The model under review builds one solid part; all positions refer to its coordinate system, in mm. A direction names the side the tool comes from. Round coordinates to 2 decimals unless told otherwise and drop trailing zeros. Write each loop counter-clockwise with the first axis right and the second up, starting at its lowest first coordinate (ties: lowest second). Pieces come first, ordered by that corner, then holes.
Item 1: Add section B-B (y = -18). State how many separate pieces and enclosed holes the cut face has, plus the area to 3 significant figures.
Item 2: Draft analysis for pull direction Z (two halves, no side actions). For faces 4 (the face through (129, 0, -48)), 5 (the face through (124.472, -12.522, -24.842)), 6 (the face through (129, -13, 0)), state which applies: +Z half, -Z half, draft (parallel to the pull), parting line (faces both ways), or undercut.
Item 3: To check wall thickness, follow L1, parallel to Z at x = 81.28, y = -17.5; L2, parallel to X at y = -2, z = -75.5; L3, parallel to X at y = -10.25, z = -74. State the ranges of each line that lie inside material, in increasing order.
Item 4: Clearance check with flat-ended pins moving along their axes: pin 1 Ø11 at (y, z) = (-16, -8) entering from +X; pin 2 Ø10 at (y, z) = (-3.5, -28.5) entering from -X; pin 3 Ø2 at (y, z) = (-18.5, -60.5) entering from +X. State where each tip first meets the part, or that it passes through.
Item 5: Machinability: for faces 1 (the face through (254, -13, -48)), 2 (the face through (254, -13, -7)), 3 (the face through (124.472, -12.522, -69.292)), which of the approach directions +Z, -Z, +X, -X, +Y, -Y give a long, thin tool a straight path to every point of the face, cutting with its end or side? Answer none if there is none.
Item 6: Add section A-A (x = 25.4). Give the boundary of the cut face in (y, z).
Item 7: Add section C-C (z = -31.5). Give the boundary of the cut face in (x, y).
Item 8: Add section D-D (z = -97). Give the boundary of the cut face in (x, y), plus the area to 3 significant figures.
```python
from build123d import *

# Parameters (mm, degrees)
F0_R     = 12.7
F1_DEPTH = 25.4


with BuildPart() as f1:
    # F0 (on Front) → F1 (new body)
    with BuildSketch(Plane.XZ):
        with BuildLine():
            Line((254, 0), (0, 0))
            Line((0, 0), (0, -127))
            Line((0, -127), (25.4, -127))
            Line((25.4, -127), (81.28, -127))
            Line((81.28, -127), (137.16, -127))
            Line((137.16, -127), (193.04, -127))
            Line((193.04, -127), (248.92, -127))
            ThreePointArc((248.92, -127), (236.4878898258, -111.7052675251), (254, -102.6602577348))
            Line((254, -102.6602577348), (254, -81.4897422652))
            ThreePointArc((254, -81.4897422652), (236.22, -69.85), (254, -58.2102577348))
            Line((254, -58.2102577348), (254, -37.0397422652))
            ThreePointArc((254, -37.0397422652), (236.22, -25.4), (254, -13.7602577348))
            Line((254, -13.7602577348), (254, 0))
        make_face()
        with BuildLine():
            ThreePointArc((38.1, -114.3), (34.3802561211, -123.2802561211), (25.4, -127))
            ThreePointArc((25.4, -127), (16.4197438789, -105.3197438789), (38.1, -114.3))
        make_face(mode=Mode.SUBTRACT)
        with BuildLine():
            ThreePointArc((93.98, -114.3), (90.2602561211, -123.2802561211), (81.28, -127))
            ThreePointArc((81.28, -127), (72.2997438789, -105.3197438789), (93.98, -114.3))
        make_face(mode=Mode.SUBTRACT)
        with Locations((25.4, -69.85)):
            Circle(F0_R, mode=Mode.SUBTRACT)
        with Locations((81.28, -69.85)):
            Circle(F0_R, mode=Mode.SUBTRACT)
        with BuildLine():
            ThreePointArc((149.86, -114.3), (146.1402561211, -123.2802561211), (137.16, -127))
            ThreePointArc((137.16, -127), (128.1797438789, -105.3197438789), (149.86, -114.3))
        make_face(mode=Mode.SUBTRACT)
        with BuildLine():
            ThreePointArc((205.74, -114.3), (202.0202561211, -123.2802561211), (193.04, -127))
            ThreePointArc((193.04, -127), (184.0597438789, -105.3197438789), (205.74, -114.3))
        make_face(mode=Mode.SUBTRACT)
        with Locations((137.16, -69.85)):
            Circle(F0_R, mode=Mode.SUBTRACT)
        with Locations((193.04, -69.85)):
            Circle(F0_R, mode=Mode.SUBTRACT)
        with Locations((25.4, -25.4)):
            Circle(F0_R, mode=Mode.SUBTRACT)
        with Locations((81.28, -25.4)):
            Circle(F0_R, mode=Mode.SUBTRACT)
        with Locations((137.16, -25.4)):
            Circle(F0_R, mode=Mode.SUBTRACT)
        with Locations((193.04, -25.4)):
            Circle(F0_R, mode=Mode.SUBTRACT)
        with BuildLine():
            ThreePointArc((38.1, -114.3), (16.4197438789, -105.3197438789), (25.4, -127))
            ThreePointArc((25.4, -127), (34.3802561211, -123.2802561211), (38.1, -114.3))
        make_face()
        with BuildLine():
            ThreePointArc((93.98, -114.3), (72.2997438789, -105.3197438789), (81.28, -127))
            ThreePointArc((81.28, -127), (90.2602561211, -123.2802561211), (93.98, -114.3))
        make_face()
        with BuildLine():
            ThreePointArc((149.86, -114.3), (128.1797438789, -105.3197438789), (137.16, -127))
            ThreePointArc((137.16, -127), (146.1402561211, -123.2802561211), (149.86, -114.3))
        make_face()
        with BuildLine():
            ThreePointArc((205.74, -114.3), (184.0597438789, -105.3197438789), (193.04, -127))
            ThreePointArc((193.04, -127), (202.0202561211, -123.2802561211), (205.74, -114.3))
        make_face()
        with BuildLine():
            Line((254, -37.0397422652), (254, -13.7602577348))
            ThreePointArc((254, -13.7602577348), (236.22, -25.4), (254, -37.0397422652))
        make_face()
        with BuildLine():
            Line((254, -81.4897422652), (254, -58.2102577348))
            ThreePointArc((254, -58.2102577348), (236.22, -69.85), (254, -81.4897422652))
        make_face()
        with BuildLine():
            Line((254, -125.9397422652), (254, -102.6602577348))
            ThreePointArc((254, -102.6602577348), (236.4878898258, -111.7052675251), (248.92, -127))
            ThreePointArc((248.92, -127), (251.5147324749, -126.7321101742), (254, -125.9397422652))
        make_face()
        with BuildLine():
            ThreePointArc((261.62, -25.4), (259.545582337, -18.4439235197), (254, -13.7602577348))
            Line((254, -13.7602577348), (254, -37.0397422652))
            ThreePointArc((254, -37.0397422652), (259.545582337, -32.3560764803), (261.62, -25.4))
        make_face()
        with BuildLine():
            ThreePointArc((261.62, -69.85), (259.545582337, -62.8939235197), (254, -58.2102577348))
            Line((254, -58.2102577348), (254, -81.4897422652))
            ThreePointArc((254, -81.4897422652), (259.545582337, -76.8060764803), (261.62, -69.85))
        make_face()
        with BuildLine():
            ThreePointArc((261.62, -114.3), (259.545582337, -107.3439235197), (254, -102.6602577348))
            Line((254, -102.6602577348), (254, -125.9397422652))
            ThreePointArc((254, -125.9397422652), (259.545582337, -121.2560764803), (261.62, -114.3))
        make_face()
        with BuildLine():
            ThreePointArc((254, -125.9397422652), (251.5147324749, -126.7321101742), (248.92, -127))
            Line((248.92, -127), (254, -127))
            Line((254, -127), (254, -125.9397422652))
        make_face()
    extrude(amount=F1_DEPTH)


solid = f1.part
```
Numbers:
1. separate pieces: 1
1. enclosed holes: 8
1. area: 28,600 mm2
2. face 4: draft
2. face 5: undercut
2. face 6: +Z half
3. L1: z = -127 to -82.55, -57.15 to -38.1, -12.7 to 0
3. L2: x = 0 to 14.03, 36.77 to 69.91, 92.65 to 125.79, 148.53 to 181.67, 204.41 to 260.29
3. L3: x = 0 to 13.4, 37.4 to 69.28, 93.28 to 125.16, 149.16 to 181.04, 205.04 to 260.92
4. pin 1: stops at x = 254
4. pin 2: stops at x = 0
4. pin 3: stops at x = 258.49
5. face 1: +X, +Y, -Y
5. face 2: +Z, +X, +Y, -Y
5. face 3: +Y, -Y
6. outline: (-25.4, -127) - (0, -127) - (0, -82.55) - (-25.4, -82.55) - close; (-25.4, -57.15) - (0, -57.15) - (0, -38.1) - (-25.4, -38.1) - close; (-25.4, -12.7) - (0, -12.7) - (0, 0) - (-25.4, 0) - close
7. outline: (0, -25.4) - (14.26, -25.4) - (14.26, 0) - (0, 0) - close; (36.54, -25.4) - (70.14, -25.4) - (70.14, 0) - (36.54, 0) - close; (92.42, -25.4) - (126.02, -25.4) - (126.02, 0) - (92.42, 0) - close; (148.3, -25.4) - (181.9, -25.4) - (181.9, 0) - (148.3, 0) - close; (204.18, -25.4) - (260.06, -25.4) - (260.06, 0) - (204.18, 0) - close
8. outline: (0, -25.4) - (254, -25.4) - (254, 0) - (0, 0) - close
8. area: 6,450 mm2
